Check sheet for the drawn part. Datum: minimum x, y, z corner. Units: mm. A direction names the side the tool comes from. Round coordinates to 2 decimals unless told otherwise and drop trailing zeros. Write each loop counter-clockwise with the first axis right and the second up, starting at its lowest first coordinate (ties: lowest second). Pieces come first, ordered by that corner, then holes. Notation, with made-up numbers: (73, 2) - (122, 2) arc R8 ccw to (122, 10) - close; hole circle Ø7 at (62, 60.25). An arc over 180 degrees is marked (long way). Return JSON: item names as keys, results as strings. Group by question number.
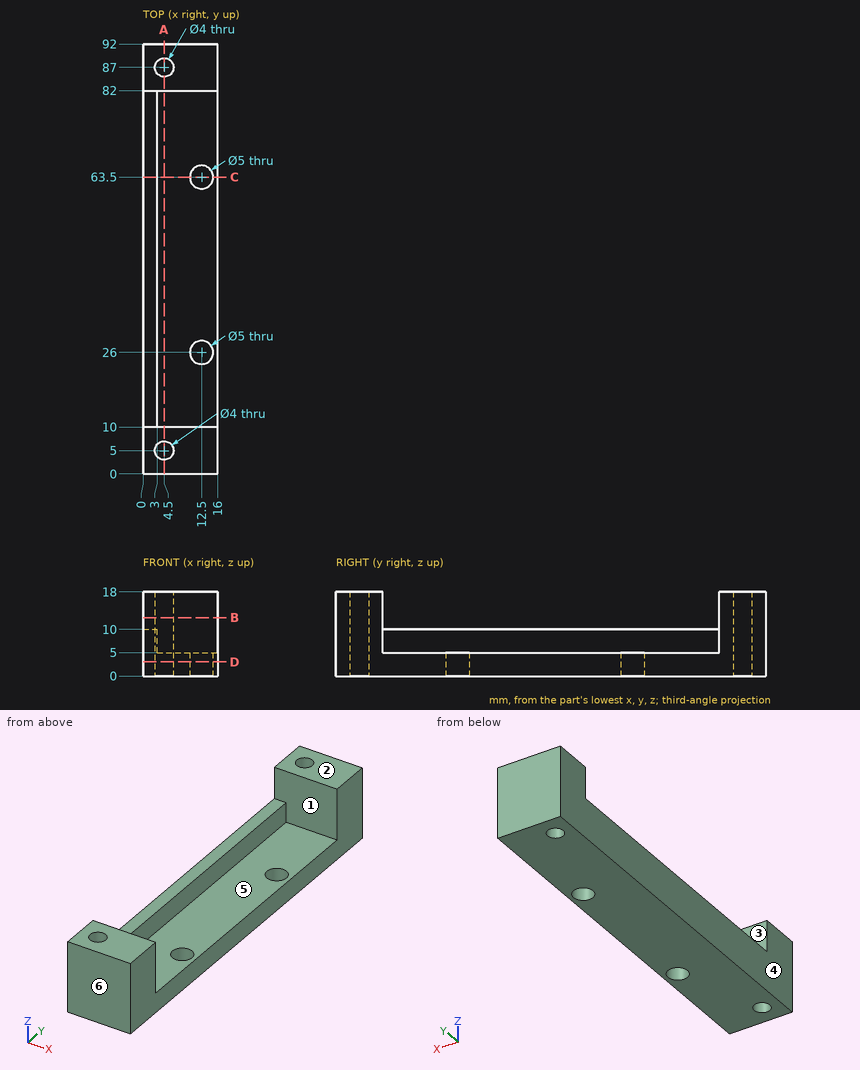
1. Tool access check on the marked faces 1 and 2. Record the directions out of +Z, -Z, +X, -X, +Y, -Y that give a thin tool (end or side, any length) a straight path to the whole face; none if there is none.
2. Mould release check, pull along Y, two halves, no side actions. Record for the marked faces 3, 4, 5 and 6: pulls with the +Y half, pulls with the -Y half, needs draft (parallel to the pull), parting line crosses it, or undercut.
3. Material ranges on line 1 along Y through (x, z) = (12.5, 3.45); line 2 along Y through (x, z) = (4.5, 10); line 3 along Y through (x, z) = (7.25, 9.5), recorded low to high.
4. Section check A-A (x = 4.5). Enter the section's corners in (y, z).
5. Section check B-B (z = 12.5). Enter the section's corners in (x, y), and give its area (3 significant figures).
6. Depth check by flat-ended pin: pin 1 Ø6.5 at (x, y) = (12.5, 63.5) entering from +Z; pin 2 Ø1.5 at (x, y) = (1.5, 60) entering from +Z; pin 3 Ø4 at (x, y) = (12.5, 26) entering from -Z. Enter the tip coordinate at first touch or a pass-through.
7. Section check C-C (y = 63.5). Enter the section's corners in (x, z), and give its area (3 significant figures).
8. Section check D-D (z = 3). Enter the section's corners in (x, y), and give its area (3 significant figures).
Result sheet:
{
 "1": {"face 1": "+Z, +X", "face 2": "+Z, +X, -X, +Y, -Y"},
 "2": {"face 3": "undercut", "face 4": "needs draft", "face 5": "undercut", "face 6": "pulls with the -Y half"},
 "3": {"line 1": "y = 0 to 23.5, 28.5 to 61, 66 to 92", "line 2": "y = 0 to 3, 7 to 10, 82 to 85, 89 to 92", "line 3": "y = 0 to 10, 82 to 92"},
 "4": {"outline": "(0, 0) - (3, 0) - (3, 18) - (0, 18) - close; (7, 0) - (85, 0) - (85, 18) - (82, 18) - (82, 5) - (10, 5) - (10, 18) - (7, 18) - close; (89, 0) - (92, 0) - (92, 18) - (89, 18) - close"},
 "5": {"outline": "(0, 0) - (16, 0) - (16, 10) - (0, 10) - close; (0, 82) - (16, 82) - (16, 92) - (0, 92) - close; hole circle Ø4 at (4.5, 5); hole circle Ø4 at (4.5, 87)", "area": "295 mm²"},
 "6": {"pin 1": "stops at z = 5", "pin 2": "stops at z = 10", "pin 3": "passes through"},
 "7": {"outline": "(0, 0) - (10, 0) - (10, 5) - (3, 5) - (3, 10) - (0, 10) - close; (15, 0) - (16, 0) - (16, 5) - (15, 5) - close", "area": "70.0 mm²"},
 "8": {"outline": "(0, 0) - (16, 0) - (16, 92) - (0, 92) - close; hole circle Ø4 at (4.5, 5); hole circle Ø4 at (4.5, 87); hole circle Ø5 at (12.5, 26); hole circle Ø5 at (12.5, 63.5)", "area": "1,410 mm²"}
}
